Build history of the part. All positions in model axes, mm. A direction names the side the tool comes from. Coordinates: 2 decimals unless noted, no trailing zeros. Loops run counter-clockwise (first coordinate to the right, second up) from the corner with the lowest first, then second, coordinate; pieces in that order, holes last.
Item 1: 3-axis set-ups, long thin cutter, end or side, ignore diameter. For faces 1 (the face through (60, 3, -47)), 2 (the face through (2, 6, 0)): which of +Z, -Z, +X, -X, +Y, -Y reach the whole face in a straight line?
Item 2: Cut at C-C (y = 128). List the corners of the cut face in (x, z) (3 decimals), and give its area (3 significant figures).
Item 3: Cut at D-D (z = 29.5). List the corners of the cut face in (x, y).
Item 4: Cut at A-A (x = 0). List the corners of the cut face in (y, z) (3 decimals).
Item 5: Cut at B-B (y = 31.5). List the corners of the cut face in (x, z) (3 decimals).
Item 6: Flat gauge pins, fed straight in: pin 1 (8 mm diameter, centred on y = 65, z = 33, fed in from +X); pin 2 (8 mm diameter, centred on x = 32, z = 65, fed in from +Y). Where does each tip first touch, or does it go through?
Item 7: Drill centre lines: line 1 along Z through (x, y) = (32, 18) (3 decimals); line 2 along X through (y, z) = (8, -42.5); line 3 along Y through (x, z) = (-51.5, -96.5). Where is each one in solid material? Low to high.
Item 8: Mould opens along Y. For faces 3 (the face through (-57.042, 103.893, 10.568)), 4 (the face through (-60, 79, 1)), 5 (the face through (-1, 0, -1)) say: released by +Y, released by -Y, zero draft, split by the parting line, or undercut.
from build123d import *

# Parameters (mm, degrees)
SKETCH1_W                 = 120
SKETCH1_H                 = 214
BOSS_EXTRUDE1_DEPTH       = 160
SHELL1_T                  = -6
SHELL1_THICKNESS_3_FACE_W = 114
SHELL1_THICKNESS_3_FACE_H = 154
SHELL1_THICKNESS_3_DEPTH  = 2.875
CUT_EXTRUDE1_REACH        = 228.824
SKETCH4_R                 = 17.5


with BuildPart() as part:
    # Sketch1 → Boss-Extrude1 (new body)
    with BuildSketch(Plane(origin=(0, 0, 0), x_dir=(1, 0, 0), z_dir=(0, 1, 0))):
        Rectangle(SKETCH1_W, SKETCH1_H)
    extrude(amount=BOSS_EXTRUDE1_DEPTH)

    # Shell1
    shell1_openings = [part.faces().sort_by_distance(p)[0] for p in [
        (0, 160, 0),
        (60, 80, 0),
    ]]
    offset(amount=SHELL1_T, openings=shell1_openings, kind=Kind.INTERSECTION)

    # Shell1 thickness 3 face (on inner face of the shell) → Shell1 thickness 3 (cut)
    with BuildSketch(Plane(origin=(3, 83, 101), x_dir=(1, 0, 0), z_dir=(0, 0, 1))):
        Rectangle(SHELL1_THICKNESS_3_FACE_W, SHELL1_THICKNESS_3_FACE_H)
    extrude(amount=SHELL1_THICKNESS_3_DEPTH, mode=Mode.SUBTRACT)

    # Sketch4 → Cut-Extrude1 (cut, up to next)
    with BuildSketch(Plane.ZY.offset(60), mode=Mode.PRIVATE) as cut_extrude1_sk1:
        with Locations((14.361495045, 120.976954776)):
            Circle(SKETCH4_R)
    cut_extrude1_tool1 = extrude(cut_extrude1_sk1.sketch, amount=-CUT_EXTRUDE1_REACH, mode=Mode.PRIVATE) & part.part
    add(cut_extrude1_tool1.solids().sort_by_distance((-60, 120.976955, 14.361495))[0], mode=Mode.SUBTRACT)


solid = part.part
Filled sheet:
1. face 1: +Z, -Z, +X, +Y, -Y
1. face 2: +X, +Y
2. outline: (-60, -107) - (60, -107) - (60, -101) - (-54, -101) - (-54, -1.667) - (-60, -1.667) - close; (-60, 30.39) - (-54, 30.39) - (-54, 103.875) - (60, 103.875) - (60, 107) - (-60, 107) - close
2. area: 2,130 mm2
3. outline: (-60, 0) - (60, 0) - (60, 6) - (-54, 6) - (-54, 112.2) - (-60, 112.2) - close; (-60, 129.76) - (-54, 129.76) - (-54, 160) - (-60, 160) - close
4. outline: (0, -107) - (160, -107) - (160, -101) - (6, -101) - (6, 103.875) - (160, 103.875) - (160, 107) - (0, 107) - close
5. outline: (-60, -107) - (60, -107) - (60, -101) - (-54, -101) - (-54, 103.875) - (60, 103.875) - (60, 107) - (-60, 107) - close
6. pin 1: stops at x = -54
6. pin 2: stops at y = 6
7. line 1: z = -107 to -101, 103.875 to 107
7. line 2: x = -60 to -54
7. line 3: y = 0 to 6
8. face 3: undercut
8. face 4: zero draft
8. face 5: released by -Y
